```python
from build123d import *

# Parameters (mm, degrees)
SKETCH1_W           = 90
SKETCH1_H           = 105
SKETCH1_R           = 1.5
BOSS_EXTRUDE1_DEPTH = 16
CHAMFER1_SIZE       = 2
SKETCH2_R           = 1.5
CUT_EXTRUDE1_DEPTH  = 10


with BuildPart() as part:
    # Sketch1 → Boss-Extrude1 (new body)
    with BuildSketch(Plane(origin=(0, 0, 0), x_dir=(1, 0, 0), z_dir=(0, 1, 0))):
        Rectangle(SKETCH1_W, SKETCH1_H)
        with Locations((-30, 44)):
            Circle(SKETCH1_R, mode=Mode.SUBTRACT)
        with Locations((30, 44)):
            Circle(SKETCH1_R, mode=Mode.SUBTRACT)
        with Locations((30, -44)):
            Circle(SKETCH1_R, mode=Mode.SUBTRACT)
        with Locations((-30, -44)):
            Circle(SKETCH1_R, mode=Mode.SUBTRACT)
        with Locations((-36, -10)):
            Circle(SKETCH1_R, mode=Mode.SUBTRACT)
        with Locations((-36, 10)):
            Circle(SKETCH1_R, mode=Mode.SUBTRACT)
        with Locations((34, 23)):
            Circle(SKETCH1_R, mode=Mode.SUBTRACT)
        with Locations((34, -23)):
            Circle(SKETCH1_R, mode=Mode.SUBTRACT)
        with BuildLine():
            Line((-15, -34), (15, -34))
            ThreePointArc((15, -34), (20.656854249, -31.656854249), (23, -26))
            Line((23, -26), (23, 26))
            ThreePointArc((23, 26), (20.656854249, 31.656854249), (15, 34))
            Line((15, 34), (-15, 34))
            ThreePointArc((-15, 34), (-20.656854249, 31.656854249), (-23, 26))
            Line((-23, 26), (-23, -26))
            ThreePointArc((-23, -26), (-20.656854249, -31.656854249), (-15, -34))
        make_face(mode=Mode.SUBTRACT)
    extrude(amount=BOSS_EXTRUDE1_DEPTH)

    # Chamfer1
    chamfer1_edges = [part.edges().sort_by_distance(p)[0] for p in [
        (-45, 16, 0),
        (0, 16, 52.5),
        (45, 16, 0),
        (0, 16, -52.5),
    ]]
    chamfer(chamfer1_edges, length=CHAMFER1_SIZE)

    # Sketch2 → Cut-Extrude1 (cut)
    with BuildSketch(Plane.XY.offset(52.5)):
        with Locations((-23, 10)):
            Circle(SKETCH2_R)
        with Locations((23, 10)):
            Circle(SKETCH2_R)
    cut_extrude1 = extrude(amount=-CUT_EXTRUDE1_DEPTH, mode=Mode.SUBTRACT)

    # Mirror1: Cut-Extrude1 across plane
    add(cut_extrude1.mirror(Plane.XY), mode=Mode.SUBTRACT)


solid = part.part
```
The model under review builds one solid part; all positions refer to its coordinate system, in mm. A direction names the side the tool comes from. Coordinates: 2 decimals unless noted, no trailing zeros. Write each loop counter-clockwise with the first axis right and the second up, starting at its lowest first coordinate (ties: lowest second). Pieces come first, ordered by that corner, then holes.
1) We need section C-C on z = 10. State the section outline as (x, y) points.
2) We need section B-B on x = 30. State the section outline as (y, z) points, then the cut area to 3 significant figures.
3) To check wall thickness, follow probe 1 along X at (y, z) = (5.5, -23); probe 2 along Z at (x, y) = (-36, 9.25); probe 3 along Z at (x, y) = (-7, 10). State the ranges of each line that lie inside material, in increasing order.
4) We need section A-A on z = -44. State the section outline as (x, y) points, then the cut area to 3 significant figures.
5) Clearance check with flat-ended pins moving along their axes: pin 1 Ø4 at (x, z) = (-36, 10) entering from -Y; pin 2 Ø1.5 at (x, y) = (-23, 9.5) entering from +Z; pin 3 Ø1.5 at (x, y) = (22.5, 10) entering from -Z. State where each tip first meets the part, or that it passes through.
6) We need section D-D on y = 2. Count the separate pieces of the cut face and the enclosed holes in it, then the cut area to 3 significant figures.
7) The part is to be moulded in two halves that separate along Z. For faces 1 (the face through (23, 8, 0)), 2 (the face through (32.89, 7.89, -24.01)), 3 (the face through (23, 10, -42.5)), 4 (the face through (-45, 7, 1)), say which applies: pulls with the +Z half, pulls with the -Z half, needs draft (parallel to the pull), parting line crosses it, or undercut.
8) Machinability: for faces 5 (the face through (-23, 10, 42.5)), 6 (the face through (-24.5, 10.07, -47.57)), 7 (the face through (20.594, 7.888, 31.719)), which of the approach directions +Z, -Z, +X, -X, +Y, -Y give a long, thin tool a straight path to every point of the face, cutting with its end or side? Answer none if there is none.
Answer list:
1. outline: (-45, 0) - (-37.5, 0) - (-37.5, 16) - (-43, 16) - (-45, 14) - close; (-34.5, 0) - (-23, 0) - (-23, 16) - (-34.5, 16) - close; (23, 0) - (45, 0) - (45, 14) - (43, 16) - (23, 16) - close
2. outline: (0, -52.5) - (14, -52.5) - (16, -50.5) - (16, -45.5) - (0, -45.5) - close; (0, -42.5) - (16, -42.5) - (16, 42.5) - (0, 42.5) - close; (0, 45.5) - (16, 45.5) - (16, 50.5) - (14, 52.5) - (0, 52.5) - close
2. area: 1,580 mm2
3. probe 1: x = -45 to -23, 23 to 32.5, 35.5 to 45
3. probe 2: z = -52.5 to -11.5, -8.5 to 8.5, 11.5 to 52.5
3. probe 3: z = -52.5 to -34, 34 to 52.5
4. outline: (-45, 0) - (-31.5, 0) - (-31.5, 16) - (-43, 16) - (-45, 14) - close; (-28.5, 0) - (28.5, 0) - (28.5, 16) - (-28.5, 16) - close; (31.5, 0) - (45, 0) - (45, 14) - (43, 16) - (31.5, 16) - close; hole circle Ø3 at (-23, 10); hole circle Ø3 at (23, 10)
4. area: 1,330 mm2
5. pin 1: stops at y = 0
5. pin 2: stops at z = 42.5
5. pin 3: stops at z = -42.5
6. separate pieces: 1
6. enclosed holes: 9
6. area: 6,320 mm2
7. face 1: undercut
7. face 2: undercut
7. face 3: pulls with the -Z half
7. face 4: needs draft
8. face 5: +Z
8. face 6: -Z
8. face 7: +Y, -Y
